from build123d import *

# Parameters (mm, degrees)
SKETCH1_R           = 9.6
SKETCH1_R_2         = 2.15
SKETCH1_R_3         = 1.6
SKETCH1_R_4         = 3.2
BOSS_EXTRUDE1_DEPTH = 3


with BuildPart() as part:
    # Sketch1 → Boss-Extrude1 (new body)
    with BuildSketch(Plane.XY):
        with BuildLine():
            Line((8, -20), (-8, -20))
            ThreePointArc((-8, -20), (-16.485281374, -16.485281374), (-20, -8))
            Line((-20, -8), (-20, 8))
            ThreePointArc((-20, 8), (-16.485281374, 16.485281374), (-8, 20))
            Line((-8, 20), (8, 20))
            ThreePointArc((8, 20), (16.485281374, 16.485281374), (20, 8))
            Line((20, 8), (20, -8))
            ThreePointArc((20, -8), (16.485281374, -16.485281374), (8, -20))
        make_face()
        Circle(SKETCH1_R, mode=Mode.SUBTRACT)
        with Locations((0, 14.5)):
            Circle(SKETCH1_R_2, mode=Mode.SUBTRACT)
        with Locations((-12.5, 0)):
            Circle(SKETCH1_R_3, mode=Mode.SUBTRACT)
        with Locations((12.5, 0)):
            Circle(SKETCH1_R_3, mode=Mode.SUBTRACT)
        with Locations((0, -14.5)):
            Circle(SKETCH1_R_2, mode=Mode.SUBTRACT)
        with Locations((10.253048327, 10.253048327)):
            Circle(SKETCH1_R_4, mode=Mode.SUBTRACT)
        with Locations((10.253048327, -10.253048327)):
            Circle(SKETCH1_R_4, mode=Mode.SUBTRACT)
        with Locations((-10.253048327, -10.253048327)):
            Circle(SKETCH1_R_4, mode=Mode.SUBTRACT)
        with Locations((-10.253048327, 10.253048327)):
            Circle(SKETCH1_R_4, mode=Mode.SUBTRACT)
    extrude(amount=BOSS_EXTRUDE1_DEPTH)


solid = part.part
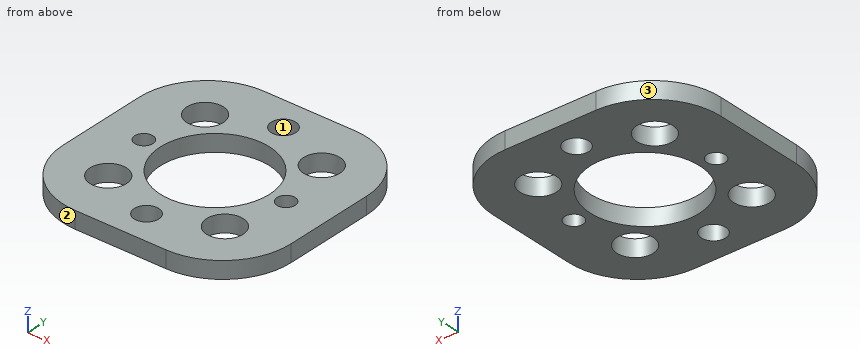
Geometry check sheet. Reference: the model listing, model coordinates, mm. Face numbers are marked on the shaded views. Round coordinates to 2 decimals unless told otherwise and drop trailing zeros. Order: outer loops, then holes, each group sorted by start corner. A loop starts at its lowest first (then second) coordinate and runs counter-clockwise, first axis right, second up. Notation, with made-up numbers: (42.25, 5.25) -> (85.25, 5.25) arc R26 cw to (85.25, 42.25) -> close; hole circle Ø1 at (83.5, 20). An arc over 180 degrees is marked (long way). Use one line per item in the form item = value.
1. Cross-section at B-B, the plane y = 0. Enter the section's corners in (x, z).
Working result:
outline = (-20, 0) -> (-14.1, 0) -> (-14.1, 3) -> (-20, 3) -> close; (-10.9, 0) -> (-9.6, 0) -> (-9.6, 3) -> (-10.9, 3) -> close; (9.6, 0) -> (10.9, 0) -> (10.9, 3) -> (9.6, 3) -> close; (14.1, 0) -> (20, 0) -> (20, 3) -> (14.1, 3) -> close
2. Cross-section at D-D, the plane z = 0.8. Count the separate pieces of the cut face and the enclosed holes in it, plus the area to 3 significant figures.
Working result:
separate_pieces = 1
enclosed_holes = 9
area = 1,010 mm^2
3. Scan lines: line 1 along Y through (x, z) = (0, 1.6); line 2 along X through (y, z) = (-1, 2.4); line 3 along X through (y, z) = (-10, 1.35). Record each from-to range of solid material in increasing order. Write a range as from..to.
Working result:
line_1 = -20..-16.65, -12.35..-9.6, 9.6..12.35, 16.65..20
line_2 = -20..-13.75, -11.25..-9.55, 9.55..11.25, 13.75..20
line_3 = -19.83..-13.44, -7.06..7.06, 13.44..19.83
4. Cross-section at A-A, the plane x = 0. Enter the section's corners in (y, z).
Working result:
outline = (-20, 0) -> (-16.65, 0) -> (-16.65, 3) -> (-20, 3) -> close; (-12.35, 0) -> (-9.6, 0) -> (-9.6, 3) -> (-12.35, 3) -> close; (9.6, 0) -> (12.35, 0) -> (12.35, 3) -> (9.6, 3) -> close; (16.65, 0) -> (20, 0) -> (20, 3) -> (16.65, 3) -> close
5. Go/stop test with flat-tipped pins: pin 1 (4 mm diameter, centred on x = 10.25, y = 10.25, fed in from -Z); pin 2 (1.5 mm diameter, centred on x = 11.5, z = 2, fed in from -Y). Record where each tip stops, or that it passes through.
Working result:
pin_1 = through
pin_2 = -19.68
6. Mould release check, pull along Y, two halves, no side actions. Record for the marked faces 1, 2 and 3: pulls with the +Y half, pulls with the -Y half, needs draft (parallel to the pull), parting line crosses it, or undercut.
Working result:
face_1 = undercut
face_2 = pulls with the -Y half
face_3 = pulls with the +Y half
7. Cross-section at C-C, the plane y = -5.5. Enter the section's corners in (x, z), plus the area to 3 significant figures.
Working result:
outline = (-20, 0) -> (-7.87, 0) -> (-7.87, 3) -> (-20, 3) -> close; (7.87, 0) -> (20, 0) -> (20, 3) -> (7.87, 3) -> close
area = 72.8 mm^2
